from build123d import *

# Parameters (mm, degrees)
CROQUIS1_R              = 3
SALIENTE_EXTRUIR1_DEPTH = 4
CROQUIS5_R              = 1.5
CORTAR_EXTRUIR4_DEPTH   = 65


with BuildPart() as part:
    # Croquis1 → Saliente-Extruir1 (new body)
    with BuildSketch(Plane(origin=(0, 0, 0), x_dir=(0, 0, -1), z_dir=(1, 0, 0))):
        with BuildLine():
            Line((0, 0), (-104.055250837, 0))
            ThreePointArc((-104.055250837, 0), (-114.055250837, 10), (-104.055250837, 20))
            Line((-104.055250837, 20), (0, 20))
            Line((0, 20), (95.944749163, 20))
            ThreePointArc((95.944749163, 20), (105.944749163, 10), (95.944749163, 0))
            Line((95.944749163, 0), (0, 0))
        make_face()
        with Locations((-4.055250837, 10)):
            Circle(CROQUIS1_R, mode=Mode.SUBTRACT)
    extrude(amount=SALIENTE_EXTRUIR1_DEPTH)

    # Croquis5 → Cortar-Extruir4 (cut)
    with BuildSketch(Plane.ZY):
        with Locations((-70.944749163, 10)):
            Circle(CROQUIS5_R)
        with Locations((-45.944749163, 10)):
            Circle(CROQUIS5_R)
        with Locations(Location((67.905250837, 10, 0), (0, 0, 180))):
            Circle(CROQUIS5_R)
        with Locations(Location((92.905250837, 10, 0), (0, 0, 180))):
            Circle(CROQUIS5_R)
    extrude(amount=-CORTAR_EXTRUIR4_DEPTH, mode=Mode.SUBTRACT)


solid = part.part
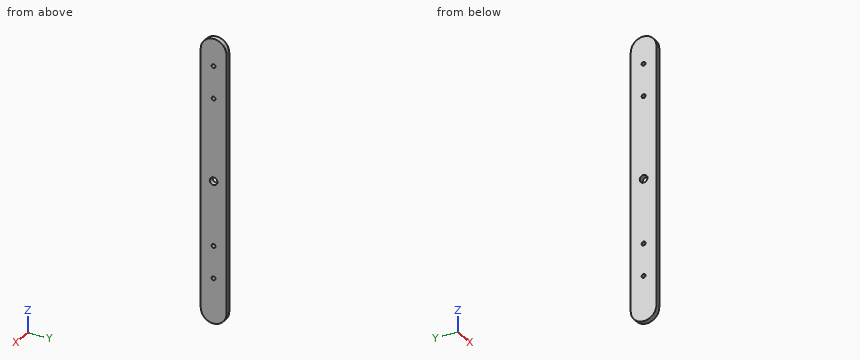
Model file for the job. Use its own axes, mm. Give positions to 0.01 mm unless a question says otherwise; leave off trailing zeros. Loops run counter-clockwise (first coordinate to the right, second up) from the corner with the lowest first, then second, coordinate; pieces in that order, holes last.
1) Wall check: line 1 (Z direction, x = 0.6, y = 11.25); line 2 (Y direction, x = 0.65, z = -45); line 3 (Z direction, x = 3.3, y = 12). Give the ranges that are in metal, low to high.
2) Saw through at A-A (x = 1.2). Write the cut outline in (y, z), plus the area to 3 significant figures.
3) Saw through at B-B (y = 16.25). Write the cut outline in (x, z), plus the area to 3 significant figures.
Answer block:
1. line 1: z = -105.87 to -71.77, -70.12 to -46.77, -45.12 to 1.33, 6.78 to 67.08, 68.73 to 92.08, 93.73 to 113.98
1. line 2: y = 0 to 8.83, 11.17 to 20
1. line 3: z = -105.74 to 1.82, 6.29 to 113.85
2. outline: (0, -95.94) arc R10 ccw to (20, -95.94) - (20, 104.06) arc R10 ccw to (0, 104.06) - close; hole circle Ø6 at (10, 4.06); hole circle Ø3 at (10, -70.94); hole circle Ø3 at (10, -45.94); hole circle Ø3 at (10, 67.91); hole circle Ø3 at (10, 92.91)
2. area: 4,260 mm2
3. outline: (0, -103.75) - (4, -103.75) - (4, 111.86) - (0, 111.86) - close
3. area: 862 mm2
